from build123d import *

# Parameters (mm, degrees)
F1_W     = 186.8932
F1_H     = 113.057654
F2_DEPTH = 25.4
F3_T     = -2.54
F0_W     = 110.6932
F0_H     = 62.257654
F4_DEPTH = 25.401


with BuildPart() as f2:
    # F1 (on Front) → F2 (new body)
    with BuildSketch(Plane.XZ):
        Rectangle(F1_W, F1_H)
    extrude(amount=F2_DEPTH)

    # F3
    f3_openings = [f2.faces().sort_by_distance(p)[0] for p in [
        (0, -25.4, 0),
    ]]
    offset(amount=F3_T, openings=f3_openings)

    # F0 (on Front) → F4 (cut, through all)
    with BuildSketch(Plane.XZ):
        Rectangle(F0_W, F0_H)
    extrude(amount=F4_DEPTH, mode=Mode.SUBTRACT)


solid = f2.part
Here's how the part is built. I have some questions about the finished solid (model axes, mm). A direction names the side the tool comes from. Coordinates: 2 decimals unless noted, no trailing zeros. Order: outer loops, then holes, each group sorted by start corner. A loop starts at its lowest first (then second) coordinate and runs counter-clockwise, first axis right, second up. Notation, with made-up numbers: M 34,-14.75 L 40,-14.75 A27 cw 40,20.25 Z; hole C -11.75,25 d5. An arc over 180 degrees is marked long. Answer as CSV lines item,"result". Start each with the question number.
1. I need wall thicknesses on line 1 (Z direction, x = -18.5, y = -2.5); line 2 (Z direction, x = 85.5, y = -4.5); line 3 (X direction, y = -3, z = -41.5). Which ranges of each line are inside material? Lowest first, please. Write a range as [from, to].
2. I want a section at C-C, the plane y = -7.25. Write out the boundary of the cut face in (x, z), and give its area (3 significant figures).
3. I want a section at B-B, the plane x = 11. Write out the boundary of the cut face in (y, z).
4. I want a section at D-D, the plane x = 66.5. Write out the boundary of the cut face in (y, z).
5. On a 3-axis mill with a long thin cutter (end or side, diameter ignored), from which of +Z, -Z, +X, -X, +Y, -Y can I reach the whole of each face in a straight line? I mean faces 4 (the flat face through (-1, -2.54, 37)), 5 (the flat face through (93.447, -13, -1)). Say none if no direction works.
6. I want a section at A-A, the plane z = -28. Write out the boundary of the cut face in (x, y), and give its area (3 significant figures).
7. We'd pull the mould along Z, two halves only. Please class faces 1 (the flat face through (0, -25.4, 55)), 2 (the flat face through (-1, -13, -56.529)), 3 (the flat face through (-90.907, -14, -1)): released by +Z, released by -Z, zero draft, split by the parting line, or undercut.
Recorded:
1,line 1,"z = [-56.53, -31.13], [31.13, 56.53]"
1,line 2,"z = [-56.53, -53.99], [53.99, 56.53]"
1,line 3,"x = [-93.45, -90.91], [90.91, 93.45]"
2,outline,"M -93.45,-56.53 L 93.45,-56.53 L 93.45,56.53 L -93.45,56.53 Z; hole M -90.91,-53.99 L 90.91,-53.99 L 90.91,53.99 L -90.91,53.99 Z"
2,area,"1,500 mm2"
3,outline,"M -25.4,-56.53 L 0,-56.53 L 0,-31.13 L -2.54,-31.13 L -2.54,-53.99 L -25.4,-53.99 Z; M -25.4,53.99 L -2.54,53.99 L -2.54,31.13 L 0,31.13 L 0,56.53 L -25.4,56.53 Z"
4,outline,"M -25.4,-56.53 L 0,-56.53 L 0,56.53 L -25.4,56.53 L -25.4,53.99 L -2.54,53.99 L -2.54,-53.99 L -25.4,-53.99 Z"
5,face 4,"-Y"
5,face 5,"+Z, -Z, +X, +Y, -Y"
6,outline,"M -93.45,-25.4 L -90.91,-25.4 L -90.91,-2.54 L -55.35,-2.54 L -55.35,0 L -93.45,0 Z; M 55.35,-2.54 L 90.91,-2.54 L 90.91,-25.4 L 93.45,-25.4 L 93.45,0 L 55.35,0 Z"
6,area,"310 mm2"
7,face 1,"zero draft"
7,face 2,"released by -Z"
7,face 3,"undercut"
